Source: CAD feature listing. Evaluate the final solid. Frame: model axes, mm. Face numbers are marked on the shaded views. A direction names the side the tool comes from. Give positions to 0.01 mm unless a question says otherwise; leave off trailing zeros. Write each loop counter-clockwise with the first axis right and the second up, starting at its lowest first coordinate (ties: lowest second). Pieces come first, ordered by that corner, then holes. Notation, with made-up numbers: (-20.75, 0.5) -> (-16.75, 0.5) arc R16 ccw to (-16.75, 29.5) -> close; hole circle Ø5 at (64.5, -32.75). An arc over 180 degrees is marked (long way). Answer as a JSON object with one key per item and string values. Group by question number.
Item 1: Section query C-C on z = 22.5. Return the cut outline in (x, y).
Item 2: Ray query, probe 1 along Z at (x, y) = (-1.5, 0); probe 2 along X at (y, z) = (1, 7); probe 3 along X at (y, z) = (0.25, 26). Return the intervals inside material, ascending. Write a range as from..to.
Item 3: Access query for the marked faces 1 and 2. Directions: +Z, -Z, +X, -X, +Y, -Y. A direction counts if a zero-diameter tool reaches every point of the face in a straight line with its end or side. Return the directions, or none.
Item 4: Section query D-D on z = 11. Return the cut outline in (x, y), plus the area to 3 significant figures.
Item 5: First-contact query: pin 1 Ø2 at (x, z) = (-0.5, 19.5) entering from -Y; pin 2 Ø6 at (x, z) = (-2.5, 25) entering from +Y; pin 3 Ø2 at (x, z) = (-2, 1.5) entering from -Y; pin 4 Ø0.6 at (x, y) = (1.5, 0) entering from -Z. Flat tips, straight axial feed; report the tip coordinate or a pass-through.
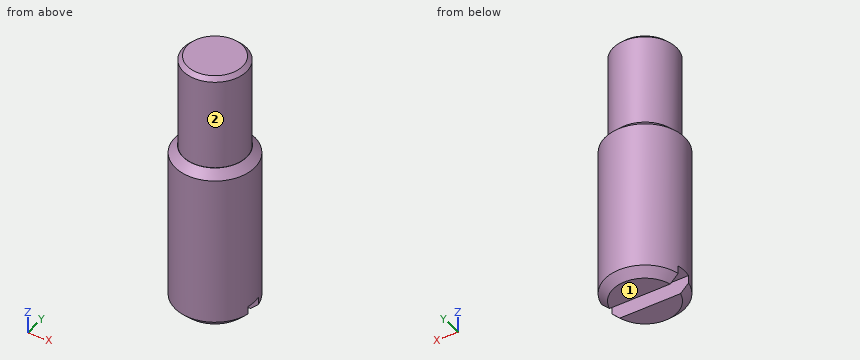
Autodesk Inventor part; units mm, degrees
ref_plane "YZ Plane" through (0, 0, 0) normal (1, 0, 0) x (0, 1, 0)
ref_plane "XZ Plane" through (0, 0, 0) normal (0, 1, 0) x (-1, 0, 0)
ref_plane "XY Plane" through (0, 0, 0) normal (0, 0, 1) x (1, 0, 0)
sketch "Sketch1" plane through (0, 0, 0) normal (0, 0, 1) x (1, 0, 0)
  circle A0 centre (0, 0) radius 5
  dimension "d0" = 10
extrude "Extrusion1" add sketch "Sketch1" along normal blind 33
sketch "Sketch2" plane through (0, 0, 33) normal (0, 0, 1) x (1, 0, 0)
  circle A0 centre (0, 0) radius 5
  circle A1 centre (0, 0) radius 3.9688
  dimension "d3" = 7.9375
extrude "Extrusion2" cut sketch "Sketch2" against normal blind 12
sketch "Sketch3" plane through (0, 0, 0) normal (0, 0, -1) x (-1, 0, 0)
  circle A0 centre (0, 0) radius 5
  line L0 (-4.899, 1) -> (4.899, 1)
  line L1 (-4.899, -1) -> (4.899, -1)
  arc A1 (-4.899, 1) -> (-4.899, -1) centre (0, 0) ccw
  arc A2 (4.899, -1) -> (4.899, 1) centre (0, 0) ccw
  dimension "d6" = 2
  dimension "d8" = 1
extrude "Extrusion3" cut sketch "Sketch3" against normal blind 2 contours A0 L1 L0
chamfer "Chamfer1" distance 1 angle 45 3 edges at (0, 5, 0) (0, -5, 0) (-5, 0, 21)
thread "Thread1"
chamfer "Chamfer2" distance 0.5 angle 45 1 edges at (-3.9688, 0, 33)
properties part number "PINO ROSCADO(25)" material "Carbon Steel"
Worked answers:
{
 "1": {"outline": "circle Ø7.94 at (0, 0)"},
 "2": {"probe 1": "2..33", "probe 2": "-4.9..4.9", "probe 3": "-3.96..3.96"},
 "3": {"face 1": "-Z, +X, -X, +Y, -Y", "face 2": "+Z"},
 "4": {"outline": "circle Ø10 at (0, 0)", "area": "78.5 mm^2"},
 "5": {"pin 1": "y = -5", "pin 2": "y = 3.97", "pin 3": "y = -4.9", "pin 4": "z = 2"}
}
